Geometry check sheet. Reference: the model listing, model coordinates, mm. A direction names the side the tool comes from. Give positions to 0.01 mm unless a question says otherwise; leave off trailing zeros. Order: outer loops, then holes, each group sorted by start corner. A loop starts at its lowest first (then second) coordinate and runs counter-clockwise, first axis right, second up. Notation, with made-up numbers: M 85.25,74 L 117.25,74 A28 cw 117.25,103 Z; hole C 69.5,47 d5. An arc over 180 degrees is marked long. Answer as CSV lines item,"result".
from build123d import *

# Parameters (mm, degrees)
F0_R           = 10
F1_DEPTH       = 16
F3_D           = 5.5
F3_CBORE_D     = 9.75
F3_CBORE_DEPTH = 5.5
F4_R           = 1


with BuildPart() as f1:
    # F0 (on Top) → F1 (new body)
    with BuildSketch(Plane.XY):
        Circle(F0_R)
    extrude(amount=F1_DEPTH)

    # F3 (through all)
    with Locations(Plane.XY.offset(16)):
        with Locations((0, 0)):
            CounterBoreHole(F3_D / 2, F3_CBORE_D / 2, F3_CBORE_DEPTH)

    # F4
    f4_edges = [f1.edges().sort_by_distance(p)[0] for p in [
        (-10, 0, 16),
        (-4.875, 0, 16),
    ]]
    fillet(f4_edges, radius=F4_R)


solid = f1.part
(1) Material ranges on line 1 (Y direction, x = 0, z = 14) (3 decimals); line 2 (Y direction, x = 0, z = 6.75); line 3 (X direction, y = -0.5, z = 15), recorded low to high.
The answers:
line 1,"y = -10 to -4.875, 4.875 to 10"
line 2,"y = -10 to -2.75, 2.75 to 10"
line 3,"x = -9.99 to -4.85, 4.85 to 9.99"
(2) Section check D-D on z = 12.5. Enter the section's corners in (x, y) (3 decimals), then the cut area to 3 significant figures.
The answers:
outline,"C 0,0 d20; hole C 0,0 d9.75"
area,"239 mm2"
(3) Gauge pin test, flat ends, axial feed: P1, Ø4, axis at x = 5.5, z = 3.5, coming from the -Y side; P2, Ø7, axis at x = 0, y = 0, coming from the +Z side; P3, Ø2, axis at x = -4.5, z = 8, coming from the +Y side. Record the tip position at first contact, or that the pin passes through.
The answers:
P1,"stops at y = -9.37"
P2,"stops at z = 10.5"
P3,"stops at y = 9.37"
(4) Draft check along Y on faces 3 (the face through (2.1, -2.1, 10.5)), 4 (the face through (-2.17, -9.76, 7.4)), 5 (the face through (2, -6, 16)). Enter one of: +Y half, -Y half, draft (parallel to the pull), parting line (faces both ways), or undercut.
The answers:
face 3,"undercut"
face 4,"parting line"
face 5,"draft"
(5) Tool access check on faces 1 (the face through (0.596, -2.685, 5.177)), 2 (the face through (-0.635, 4.834, 12.782)). Record the directions out of +Z, -Z, +X, -X, +Y, -Y that give a thin tool (end or side, any length) a straight path to the whole face; none if there is none.
The answers:
face 1,"+Z, -Z"
face 2,"+Z"
(6) Section check C-C on z = 5.5. Enter the section's corners in (x, y).
The answers:
outline,"C 0,0 d20; hole C 0,0 d5.5"
(7) Section check A-A on x = 0. Enter the section's corners in (y, z) (3 decimals).
The answers:
outline,"M -10,0 L -2.75,0 L -2.75,10.5 L -4.875,10.5 L -4.875,15 A1 ccw -5.875,16 L -9,16 A1 ccw -10,15 Z; M 2.75,0 L 10,0 L 10,15 A1 ccw 9,16 L 5.875,16 A1 ccw 4.875,15 L 4.875,10.5 L 2.75,10.5 Z"
